```python
from build123d import *

# Parameters (mm, degrees)
BOSS_EXTRUDE1_DEPTH      = 40
BOSS_EXTRUDE2_REACH      = 151.282
BOSS_EXTRUDE2_END_RADIUS = 39.99999999999999
BOSS_EXTRUDE2_START      = 80
SKETCH2_W                = 50.00000000000001
SKETCH2_H                = 10
CUT_EXTRUDE6_START       = -10
CUT_EXTRUDE6_DEPTH       = 10
BOSS_EXTRUDE4_DEPTH      = 102
CUT_EXTRUDE7_REACH       = 140.939
BOSS_EXTRUDE5_DEPTH      = 10
CUT_EXTRUDE8_START       = -10
CUT_EXTRUDE8_DEPTH       = 10
CUT_EXTRUDE9_REACH       = 133.773
SKETCH9_R                = 8.000000000000012
BOSS_EXTRUDE6_DEPTH      = 5


with BuildPart() as part:
    # Sketch1 → Boss-Extrude1 (new body)
    with BuildSketch(Plane.XY):
        with BuildLine():
            Line((-39.999999999999986, 0), (-30, 0))
            ThreePointArc((-30, 0), (1.84e-15, 30), (30, 0))
            Line((30, 0), (39.99999999999999, 0))
            ThreePointArc((39.99999999999999, 0), (2.45e-15, 39.99999999999999), (-39.999999999999986, 0))
        make_face()
    extrude(amount=-BOSS_EXTRUDE1_DEPTH)

    # Boss-Extrude2: up to this cylinder (the profile starts outside it)
    boss_extrude2_end = Plane(origin=(0, 0, -25), z_dir=(0, 0, 1)) * Cylinder(BOSS_EXTRUDE2_END_RADIUS, 383.564, mode=Mode.PRIVATE)
    # Sketch2 → Boss-Extrude2 (add, up to the surface)
    with BuildSketch(Plane(origin=(0, 0, 0), x_dir=(0, 0, -1), z_dir=(1, 0, 0)).offset(BOSS_EXTRUDE2_START), mode=Mode.PRIVATE) as boss_extrude2_sk1:
        with Locations((25.000000000000004, 5)):
            Rectangle(SKETCH2_W, SKETCH2_H)
    boss_extrude2_tool1 = extrude(boss_extrude2_sk1.sketch, amount=-BOSS_EXTRUDE2_REACH, mode=Mode.PRIVATE) - boss_extrude2_end
    boss_extrude2 = boss_extrude2_tool1.solids().sort_by_distance((80, 5, -25))[0]
    add(boss_extrude2)

    # Sketch3 → Cut-Extrude6 (cut)
    with BuildSketch(Plane(origin=(0, 10, 0), x_dir=(1, 0, 0), z_dir=(0, 1, 0)).offset(CUT_EXTRUDE6_START)):
        with BuildLine():
            ThreePointArc((43.72983346207417, 5.000000000000001), (40.194299556141424, 3.5355339059327426), (38.72983346207416, 0))
            Line((38.72983346207416, 0), (80, 0))
            Line((80, 0), (80, 25.000000000000007))
            ThreePointArc((80, 25.000000000000007), (74.14213562373095, 10.857864376269053), (60, 5))
            Line((60, 5.000000000000001), (43.72983346207417, 5))
        make_face()
        with BuildLine():
            Line((80, 50), (38.72983346207416, 50))
            ThreePointArc((38.72983346207416, 50), (40.194299556141424, 46.464466094067255), (43.72983346207417, 45))
            Line((43.72983346207417, 45), (60, 45))
            ThreePointArc((60, 45), (74.14213562373095, 39.14213562373095), (80, 25.000000000000007))
            Line((80, 25.000000000000007), (80, 50))
        make_face()
    cut_extrude6 = extrude(amount=CUT_EXTRUDE6_DEPTH, mode=Mode.SUBTRACT)

    # Mirror1: Boss-Extrude2, Cut-Extrude6 across plane
    add(boss_extrude2.mirror(Plane(origin=(0, 0, 0), x_dir=(0, 0, 1), z_dir=(1, 0, 0))))
    add(cut_extrude6.mirror(Plane(origin=(0, 0, 0), x_dir=(0, 0, 1), z_dir=(1, 0, 0))), mode=Mode.SUBTRACT)

    # Sketch4 → Boss-Extrude4 (add)
    with BuildSketch(Plane(origin=(0, 0, 0), x_dir=(1, 0, 0), z_dir=(0, 1, 0))):
        Polygon((-39.99999999999999, 40), (39.99999999999999, 40), (39.99999999999999, 50.00000000000003), (-39.99999999999999, 50), align=None)
    extrude(amount=BOSS_EXTRUDE4_DEPTH)

    # Sketch6 → Cut-Extrude7 (cut, up to next)
    with BuildSketch(Plane(origin=(-1.735e-14, 0, -50.000000000000014), x_dir=(-1, 0, 3.5e-16), z_dir=(-3.5e-16, 0, -1)), mode=Mode.PRIVATE) as cut_extrude7_sk1:
        with BuildLine():
            Line((-30, 0), (30, 0))
            ThreePointArc((30, 0), (1.84e-15, 30), (-30, 0))
        make_face()
    cut_extrude7_tool1 = extrude(cut_extrude7_sk1.sketch, amount=-CUT_EXTRUDE7_REACH, mode=Mode.PRIVATE) & part.part
    add(cut_extrude7_tool1.solids().sort_by_distance((0, 12.732395, -50))[0], mode=Mode.SUBTRACT)

    # Sketch7 → Boss-Extrude5 (add)
    with BuildSketch(Plane.XY.offset(-40)):
        with BuildLine():
            Line((-25, 102), (-16, 102))
            ThreePointArc((-16, 102), (-2.94e-15, 86), (16, 102))
            Line((16, 102), (25, 102))
            ThreePointArc((25, 102), (-4.59e-15, 77), (-25, 102))
        make_face()
    extrude(amount=BOSS_EXTRUDE5_DEPTH)

    # Sketch8 → Cut-Extrude8 (cut)
    with BuildSketch(Plane.XY.offset(-40).offset(CUT_EXTRUDE8_START)):
        with BuildLine():
            Line((16, 102), (-16, 101.99999999999989))
            ThreePointArc((-16, 101.99999999999989), (5.782e-14, 85.99999999999994), (16, 102))
        make_face()
        Polygon((-25, 102), (-39.99999999999999, 102), (-39.99999999999999, 10), align=None)
        Polygon((25.000000000000004, 102), (39.99999999999999, 102), (39.99999999999999, 9.999999999999998), align=None)
    extrude(amount=CUT_EXTRUDE8_DEPTH, mode=Mode.SUBTRACT)

    # Sketch9 → Cut-Extrude9 (cut, up to next)
    with BuildSketch(Plane(origin=(0, 10, 0), x_dir=(1, 0, 0), z_dir=(0, 1, 0)), mode=Mode.PRIVATE) as cut_extrude9_sk1:
        with Locations(Location((60, 25, 0), (0, 0, 270))):
            Circle(SKETCH9_R)
    cut_extrude9_tool1 = extrude(cut_extrude9_sk1.sketch, amount=-CUT_EXTRUDE9_REACH, mode=Mode.PRIVATE) & part.part
    cut_extrude9 = cut_extrude9_tool1.solids().sort_by_distance((60, 10, -25))[0]
    add(cut_extrude9, mode=Mode.SUBTRACT)

    # Mirror2: Cut-Extrude9 across plane
    add(cut_extrude9.mirror(Plane(origin=(0, 0, 0), x_dir=(0, 0, 1), z_dir=(1, 0, 0))), mode=Mode.SUBTRACT)

    # Sketch11 → Boss-Extrude6 (add, symmetric)
    with BuildSketch(Plane(origin=(0, 0, 0), x_dir=(0, 0, -1), z_dir=(1, 0, 0))):
        Polygon((0, 30), (0, 39.99999999999999), (30, 76.99999999999999), (30, 86), (40, 86), (40, 30), align=None)
    extrude(amount=BOSS_EXTRUDE6_DEPTH, both=True)


solid = part.part
```
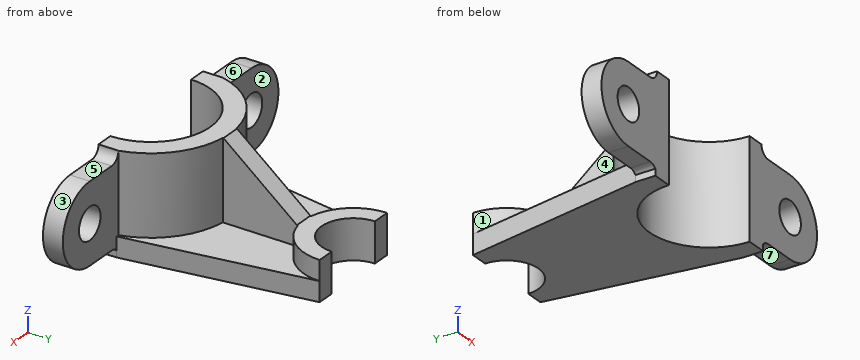
The model under review builds one solid part; all positions refer to its coordinate system, in mm. Face numbers are marked on the shaded views. A direction names the side the tool comes from. Give positions to 0.01 mm unless a question says otherwise; leave off trailing zeros. Write each loop counter-clockwise with the first axis right and the second up, starting at its lowest first coordinate (ties: lowest second). Pieces come first, ordered by that corner, then holes. Notation, with made-up numbers: M 64,89 L 118,89 A26 ccw 118,119 Z; hole C 41.5,-39.75 d7. An arc over 180 degrees is marked long. Write each question's results on one line, items separated by ' | '. Start each with the question number.
1. We need section A-A (z = -25). Write out the cut boundary in (x, y), and give its area (3 significant figures).
2. For probe 1 along X at (y, z) = (2, -25); probe 2 along X at (y, z) = (4, -25); probe 3 along Y at (x, z) = (-71, -40.5), list the stretches that pass through material, from the lowest coordinate up. Write a range as [from, to].
3. We need section C-C (x = 0). Write out the cut boundary in (y, z).
4. Mouldability with a two-part tool opening along Y and no side actions: class the marked faces 1, 2 and 3 as released by +Y, released by -Y, zero draft, split by the parting line, or undercut.
5. We need section B-B (y = 88). Write out the cut boundary in (x, z), and give its area (3 significant figures).
6. We need section D-D (x = 56). Write out the cut boundary in (y, z).
7. For the marked faces 4, 5, 6 and 7, list the 3-axis set-ups (+Z, -Z, +X, -X, +Y, -Y) from which the entire face can be reached by the end or side of a thin tool; tool diameter is ignored.
8. Insertion check: pin 1 Ø5 at (x, y) = (-49.5, 7) entering from -Z; pin 2 Ø1 at (y, z) = (5, -49) entering from -X; pin 3 Ø1.5 at (x, y) = (-18.5, 81) entering from +Z. Each pin has a flat end and moves straight along its axis. Give the tip position at first contact, or say it passes through.
Results found:
1) outline: M -80,0 L -68,0 L -68,10 L -80,10 Z; M -52,0 L -30,0 A30 cw 30,0 L 52,0 L 52,10 L 38.73,10 A40 ccw 5,39.69 L 5,70.83 L -5,70.83 L -5,39.69 A40 ccw -38.73,10 L -52,10 Z; M 68,0 L 80,0 L 80,10 L 68,10 Z | area: 1,900 mm^2
2) probe 1: x = [-80, -68], [-52, -29.93], [29.93, 52], [68, 80] | probe 2: x = [-80, -68], [-52, -29.73], [29.73, 52], [68, 80] | probe 3: y = [0, 10]
3) outline: M 30,-50 L 86,-50 L 86,-30 L 77,-30 L 40,0 L 30,0 Z
4) face 1: undercut | face 2: released by +Y | face 3: zero draft
5) outline: M -27.28,-50 L -7.75,-50 L -7.75,-30 L -20.71,-30 L -20.71,-40 L -27.28,-40 Z; M 7.75,-50 L 27.28,-50 L 27.28,-40 L 20.71,-40 L 20.71,-30 L 7.75,-30 Z | area: 650 mm^2
6) outline: M 0,-45 L 10,-45 L 10,-31.93 L 0,-31.93 Z; M 0,-18.07 L 10,-18.07 L 10,-5 L 0,-5 Z
7) face 4: +Z, -X | face 5: +Z, +X, +Y, -Y | face 6: +Z, -X, +Y, -Y | face 7: -Z, +X, +Y, -Y
8) pin 1: stops at z = -45 | pin 2: stops at x = -40 | pin 3: stops at z = -40
